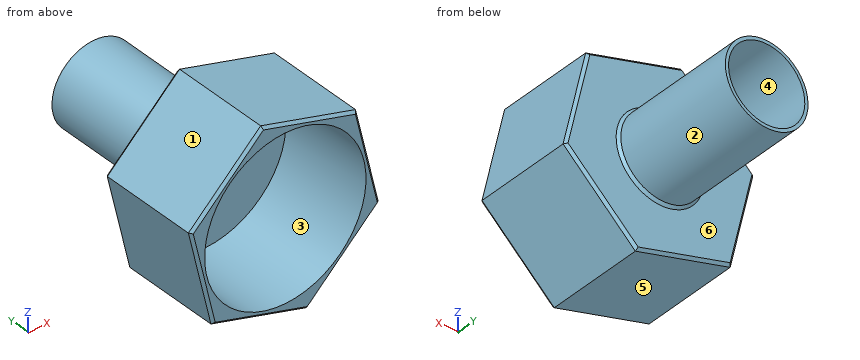
from build123d import *

# Parameters (mm, degrees)
SKETCH_1_R          = 3.253
EXTRUDE_1_DEPTH     = 10
SKETCH_2_R          = 3
CUT_EXTRUDE_1_DEPTH = 10
EXTRUDE_2_DEPTH     = 8
CHAMFER_2_SIZE      = 0.2
SKETCH_6_R          = 6.35
CUT_EXTRUDE_3_DEPTH = 7.5
SCALE_1_SCALE       = 1.703703703


with BuildPart() as part:
    # 草图1 → 凸台-拉伸1 (new body)
    with BuildSketch(Plane(origin=(0, 0, 0), x_dir=(1, 0, 0), z_dir=(0, 1, 0))):
        with Locations(Location((0, 0, 0), (0, 0, 270))):
            Circle(SKETCH_1_R)
    extrude(amount=EXTRUDE_1_DEPTH)

    # 草图2 → 切除-拉伸1 (cut)
    with BuildSketch(Plane.XZ):
        with Locations(Location((0, 0, 0), (0, 0, 270))):
            Circle(SKETCH_2_R)
    extrude(amount=-CUT_EXTRUDE_1_DEPTH, mode=Mode.SUBTRACT)

    # 草图3 → 凸台-拉伸2 (add)
    with BuildSketch(Plane.XZ):
        Polygon((1.774601568, -7.589518382), (7.460016506, -2.257909151), (5.685414937, 5.331609231), (-1.774601568, 7.589518382), (-7.460016506, 2.257909151), (-5.685414937, -5.331609231), align=None)
    extrude(amount=EXTRUDE_2_DEPTH)

    # 倒角2
    chamfer_2_edges = [part.edges().sort_by_distance(p)[0] for p in [
        (0, 0, -3.253),
        (-1.955406684, 0, -6.460563807),
        (4.617309037, 0, -4.923713767),
        (6.572715721, 0, 1.53685004),
        (1.955406684, 0, 6.460563807),
        (-4.617309037, 0, 4.923713767),
        (-6.572715721, 0, -1.53685004),
        (-1.955406684, -8, -6.460563807),
        (4.617309037, -8, -4.923713767),
        (6.572715721, -8, 1.53685004),
        (1.955406684, -8, 6.460563807),
        (-4.617309037, -8, 4.923713767),
        (-6.572715721, -8, -1.53685004),
    ]]
    chamfer(chamfer_2_edges, length=CHAMFER_2_SIZE)

    # 草图6 → 切除-拉伸3 (cut)
    with BuildSketch(Plane.XZ.offset(8)):
        with Locations(Location((0, 0, 0), (0, 0, 270))):
            Circle(SKETCH_6_R)
    extrude(amount=-CUT_EXTRUDE_3_DEPTH, mode=Mode.SUBTRACT)


with BuildPart() as part_1:
    # 缩放比例1: scaled about (0, -2.097517818, 0)
    add(part.part.scale(SCALE_1_SCALE).moved(Location((0, 1.476031056, 0))))


solid = part_1.part
Geometry: final body of the model. Coordinates: model frame, mm. Face numbers are marked on the shaded views. A direction names the side the tool comes from. Round coordinates to 2 decimals unless told otherwise and drop trailing zeros. Loops run counter-clockwise (first coordinate to the right, second up) from the corner with the lowest first, then second, coordinate; pieces in that order, holes last. Notation, with made-up numbers: (-26.5, -38.5) - (-8.5, -38.5) arc R26 ccw to (-8.5, 0.5) - close; hole circle Ø8 at (71, 84.25). An arc over 180 degrees is marked (long way). Write each question's results on one line, items separated by ' | '. Start each with the question number.
1) Cut plane C-C on z = 0. Return loops of the section in (x, y).
2) Access query for the marked faces 1, 2 and 3. Directions: +Z, -Z, +X, -X, +Y, -Y. A direction counts if a zero-diameter tool reaches every point of the face in a straight line with its end or side. Return the directions, or none.
3) Cut plane A-A on y = -7. Return loops of the section in (x, z), then the cut area to 3 significant figures.
4) First-contact query: P1, Ø4, axis at x = -3, y = 12, coming from the +Z side; P2, Ø5, axis at x = -1, z = 1, coming from the +Y side; P3, Ø4, axis at x = 7, y = -4.5, coming from the +Z side. Flat tips, straight axial feed; report the tip coordinate or a pass-through.
5) Cut plane B-B on x = 0. Return loops of the section in (y, z).
6) Mould query, pull axis X, two halves, no side actions, for the marked faces 4, 5 and 6. Classes: released by +X, released by -X, zero draft, split by the parting line, or undercut.
7) Cut plane D-D on y = 9. Return loops of the section in (x, z), then the cut area to 3 significant figures.
8) Line query: probe 1 along X at (y, z) = (12, 0); probe 2 along X at (y, z) = (-3.5, -3.5); probe 3 along Z at (x, y) = (-6.5, -4). Output: solid intervals per line, ascending. Write a range as [from, to].
Verdict:
1) outline: (-11.81, -11.81) - (-11.46, -12.15) - (-10.82, -12.15) - (-10.82, 0.62) - (10.82, 0.62) - (10.82, -12.15) - (11.46, -12.15) - (11.81, -11.81) - (11.81, 1.14) - (11.46, 1.48) - (5.88, 1.48) - (5.54, 1.82) - (5.54, 18.51) - (5.11, 18.51) - (5.11, 1.48) - (-5.11, 1.48) - (-5.11, 18.51) - (-5.54, 18.51) - (-5.54, 1.82) - (-5.88, 1.48) - (-11.46, 1.48) - (-11.81, 1.14) - close
2) face 1: +Z, -X, +Y, -Y | face 2: +Y | face 3: -Y
3) outline: (-12.71, 3.85) - (-9.69, -9.08) - (3.02, -12.93) - (12.71, -3.85) - (9.69, 9.08) - (-3.02, 12.93) - close; hole circle Ø21.64 at (0, 0) | area: 90.4 mm2
4) P1: stops at z = 5.45 | P2: stops at y = 1.48 | P3: stops at z = 10.5
5) outline: (-12.15, -11.66) - (-11.81, -12.02) - (1.14, -12.02) - (1.48, -11.66) - (1.48, -5.88) - (1.82, -5.54) - (18.51, -5.54) - (18.51, -5.11) - (1.48, -5.11) - (1.48, 5.11) - (18.51, 5.11) - (18.51, 5.54) - (1.82, 5.54) - (1.48, 5.88) - (1.48, 11.66) - (1.14, 12.02) - (-11.81, 12.02) - (-12.15, 11.66) - (-12.15, 10.82) - (0.62, 10.82) - (0.62, -10.82) - (-12.15, -10.82) - close
6) face 4: undercut | face 5: released by -X | face 6: zero draft
7) outline: circle Ø11.08 at (0, 0); hole circle Ø10.22 at (0, 0) | area: 14.4 mm2
8) probe 1: x = [-5.54, -5.11], [5.11, 5.54] | probe 2: x = [-10.99, -10.24], [10.24, 12.63] | probe 3: z = [-10.05, -8.65], [8.65, 9.67]
